```python
from build123d import *

# Parameters (mm, degrees)
F0_R        = 3.2004
F0_R_2      = 6.2992
F0_R_3      = 5.08
F0_R_4      = 11.2395
F1_DEPTH    = 31.75
F2_W        = 12.7
F2_H        = 5.1071889116
F3_DEPTH    = 31.75
F4_T1_DEPTH = 31.75
F5_R        = 1.27
F6_R        = 2.9845
F7_DEPTH    = 25.4


# Not quite as in the source:
# - a fillet or chamfer that OpenCascade refuses, or shapes differently, is made with other operations: its cross-section is extruded or revolved along the edge and cut away or added


with BuildPart() as f1:
    # F0 (on Top) → F1 (new body)
    with BuildSketch(Plane.XY):
        with BuildLine():
            Line((-5.159375, 19.9821734518), (-40.878125, 10.7596318587))
            ThreePointArc((-40.878125, 10.7596318587), (-49.2125, 0), (-40.878125, -10.7596318587))
            Line((-40.878125, -10.7596318587), (-5.159375, -19.9821734518))
            ThreePointArc((-5.159375, -19.9821734518), (0, -20.6375), (5.159375, -19.9821734518))
            Line((5.159375, -19.9821734518), (40.878125, -10.7596318587))
            ThreePointArc((40.878125, -10.7596318587), (49.2125, 0), (40.878125, 10.7596318587))
            Line((40.878125, 10.7596318587), (5.159375, 19.9821734518))
            ThreePointArc((5.159375, 19.9821734518), (0, 20.6375), (-5.159375, 19.9821734518))
        make_face()
        with Locations((-12.7, -12.7)):
            Circle(F0_R, mode=Mode.SUBTRACT)
        with Locations((12.7, -12.7)):
            Circle(F0_R, mode=Mode.SUBTRACT)
        with Locations((-38.1, 0)):
            Circle(F0_R_2, mode=Mode.SUBTRACT)
        with Locations((-19.05, 0)):
            Circle(F0_R_3, mode=Mode.SUBTRACT)
        with Locations((-12.7, 12.7)):
            Circle(F0_R, mode=Mode.SUBTRACT)
        Circle(F0_R_4, mode=Mode.SUBTRACT)
        with Locations((19.05, 0)):
            Circle(F0_R_3, mode=Mode.SUBTRACT)
        with Locations((38.1, 0)):
            Circle(F0_R_2, mode=Mode.SUBTRACT)
        with Locations((12.7, 12.7)):
            Circle(F0_R, mode=Mode.SUBTRACT)
    extrude(amount=F1_DEPTH)

    # F2 (on face) → F3 (join)
    with BuildSketch(Plane.XY.offset(31.75)):
        with Locations((0, 20.7509055442)):
            Rectangle(F2_W, F2_H)
    extrude(amount=-F3_DEPTH)

    # F4: fillet of radius 12.7 on 2 edges, made by hand

    # F4_s2 → F4_t1 (join)
    with BuildSketch(Plane.XY):
        with BuildLine():
            ThreePointArc((-13.9630832797, 17.7090657484), (-9.6168370541, 19.7724670423), (-6.35, 23.3045))
            Line((-6.35, 23.3045), (-6.35, 19.6747553987))
            Line((-6.35, 19.6747553987), (-13.9630832797, 17.7090657484))
        make_face()
        with BuildLine():
            ThreePointArc((13.9630832797, 17.7090657484), (9.6168370541, 19.7724670423), (6.35, 23.3045))
            Line((6.35, 23.3045), (6.35, 19.6747553987))
            Line((6.35, 19.6747553987), (13.9630832797, 17.7090657484))
        make_face()
    extrude(amount=F4_T1_DEPTH)

    # F5
    f5_edges = [f1.edges().sort_by_distance(p)[0] for p in [
        (-6.35, 23.3045, 15.875),
        (6.35, 23.3045, 15.875),
    ]]
    fillet(f5_edges, radius=F5_R)

    # F6 (on face) → F7 (cut)
    with BuildSketch(Plane(origin=(0, 23.3045, 0), x_dir=(-1, 0, 0), z_dir=(0, 1, 0))):
        with Locations((0, 15.875)):
            Circle(F6_R)
    extrude(amount=-F7_DEPTH, mode=Mode.SUBTRACT)


solid = f1.part
```
Build history of the part. All positions in model axes, mm. A direction names the side the tool comes from. Give positions to 0.01 mm unless a question says otherwise; leave off trailing zeros. Loops run counter-clockwise (first coordinate to the right, second up) from the corner with the lowest first, then second, coordinate; pieces in that order, holes last. Notation, with made-up numbers: (47.25, 75.25) - (90.25, 75.25) arc R16 ccw to (90.25, 103.25) - close; hole circle Ø10 at (63, 60.5). An arc over 180 degrees is marked (long way). Use a Markdown table: item, result.
(1) Pull direction X, two halves, no side cores. Call faces 3 (the face through (-10.98, -10, 15.65)), 4 (the face through (-0.073, -20.637, 15.653)), 5 (the face through (-27.232, 14.283, 15.653)): +X half, -X half, draft (parallel to the pull), parting line (faces both ways), or undercut.
Taken from the geometry:
| item | result |
|---|---|
| face 3 | undercut |
| face 4 | parting line |
| face 5 | -X half |
(2) Band-saw the part on D-D (x = -22). Give the cut face in (y, z).
Taken from the geometry:
| item | result |
|---|---|
| outline | (-15.63, 0) - (-4.14, 0) - (-4.14, 31.75) - (-15.63, 31.75) - close; (4.14, 0) - (15.63, 0) - (15.63, 31.75) - (4.14, 31.75) - close |
(3) Band-saw the part on B-B (x = 0). Give the cut face in (y, z), and give its area (3 significant figures).
Taken from the geometry:
| item | result |
|---|---|
| outline | (-20.64, 0) - (-11.24, 0) - (-11.24, 31.75) - (-20.64, 31.75) - close; (11.24, 0) - (23.3, 0) - (23.3, 12.89) - (11.24, 12.89) - close; (11.24, 18.86) - (23.3, 18.86) - (23.3, 31.75) - (11.24, 31.75) - close |
| area | 609 mm2 |
(4) Which spindle directions (+Z, -Z, +X, -X, +Y, -Y) get a long thin tool onto all of the face, cutting with end or side? Do faces 1 (the face through (-9.93, 19.55, 15.65)), 2 (the face through (0.389, 17.155, 18.834)). Say none if no direction does.
Taken from the geometry:
| item | result |
|---|---|
| face 1 | +Z, -Z, -X, +Y |
| face 2 | +Y |
(5) Drop flat-ended pins along their axis: pin 1 Ø5 at (x, z) = (7.5, 23) entering from -Y; pin 2 Ø5 at (x, y) = (12.7, 12.7) entering from -Z; pin 3 Ø10 at (x, z) = (-37, 27) entering from -Y; pin 4 Ø5 at (x, z) = (33.5, 6.5) entering from +Y. Give the stop position or say it passes through.
Taken from the geometry:
| item | result |
|---|---|
| pin 1 | y = -20.02 |
| pin 2 | through |
| pin 3 | y = -13.05 |
| pin 4 | y = 13.31 |
(6) Wall check: line 1 along Y through (x, z) = (12.7, 8); line 2 along Y through (x, z) = (-15.5, 30); line 3 along X through (y, z) = (1, 14). Give the ranges that are in metal, low to high.
Taken from the geometry:
| item | result |
|---|---|
| line 1 | -18.04 to -15.9, -9.5 to 9.5, 15.9 to 18.11 |
| line 2 | -17.31 to -14.25, -11.15 to -3.63, 3.63 to 11.15, 14.25 to 17.31 |
| line 3 | -49.17 to -44.32, -31.88 to -24.03, -14.07 to -11.19, 11.19 to 14.07, 24.03 to 31.88, 44.32 to 49.17 |
(7) Band-saw the part on A-A (z = 5). Give the number of separate pieces and of enclosed holes in the cut face, and give its area (3 significant figures).
Taken from the geometry:
| item | result |
|---|---|
| separate pieces | 1 |
| enclosed holes | 9 |
| area | 2,000 mm2 |
